Can you work these out from the model? Positions are in its coordinate system, mm. Face numbers are marked on the shaded views. A direction names the side the tool comes from. Give positions to 0.01 mm unless a question says otherwise; leave off trailing zeros. Order: outer loops, then holes, each group sorted by start corner. A loop starts at its lowest first (then second) coordinate and runs counter-clockwise, first axis right, second up.
Item 1: I want a section at B-B, the plane x = 0. Write out the boundary of the cut face in (y, z), then the cut area to 3 significant figures.
Item 2: Which directions (+Z, -Z, +X, -X, +Y, -Y) give clear straight access to the entire face, cutting with the end or side of a thin tool? Please do the marked faces 1, 2, 3 and 4.
Item 3: I'm going to push flat-ended pins straight in: pin 1 Ø1 at (x, y) = (1, 77.5) entering from -Z; pin 2 Ø4.5 at (x, y) = (0, 47) entering from -Z; pin 3 Ø3 at (x, z) = (1, -37.5) entering from +Y; pin 4 Ø3 at (x, y) = (-0.5, 33) entering from +Z. Where does each tip first touch, or does it pass through?
Item 4: I want a section at A-A, the plane y = 65.5. Write out the boundary of the cut face in (x, z).
Item 5: If I drill on line 1 along Z through (x, y) = (3.75, 36); line 2 along Y through (x, z) = (0, 30.9); line 3 along Y through (x, z) = (-2, -23.5), over which ranges is the centre line in solid material (lowest first)?
Item 6: I want a section at D-D, the plane z = 11. Write out the boundary of the cut face in (x, y), then the cut area to 3 significant figures.
Item 7: I want a section at C-C, the plane y = 47. Write out the boundary of the cut face in (x, z).
Item 8: If we mould it in two halves opening along Z, with no side actions, what happens to the marked faces 5, 6 and 7? For each: +Z half, -Z half, draft (parallel to the pull), parting line (faces both ways), or undercut.
```python
from build123d import *

# Parameters (mm, degrees)
BOSS_EXTRUDE1_DEPTH      = 5
BOSS_EXTRUDE1_DEPTH_BACK = 5
SKETCH2_R                = 2.5
CUT_EXTRUDE1_DEPTH       = 124.328828747


with BuildPart() as part:
    # Sketch1 → Boss-Extrude1 (new, two sides: drawn at the far end of the back side and taken through both)
    with BuildSketch(Plane(origin=(0, 0, 0), x_dir=(0, 0, -1), z_dir=(1, 0, 0)).offset(-BOSS_EXTRUDE1_DEPTH_BACK)):
        Polygon((-33, 3), (-33, 97), (33, 97), (33, 3), (43, 3), (43, 0), (33, 0), (28, 0), (28, 92), (-28, 92), (-28, 0), (-33, 0), (-43, 0), (-43, 3), align=None)
    extrude(amount=BOSS_EXTRUDE1_DEPTH + BOSS_EXTRUDE1_DEPTH_BACK)

    # Sketch2 → Cut-Extrude1 (cut, through all)
    with BuildSketch(Plane.XY.offset(33)):
        with Locations((0, 47)):
            Circle(SKETCH2_R)
    extrude(amount=-CUT_EXTRUDE1_DEPTH, mode=Mode.SUBTRACT)


solid = part.part
```
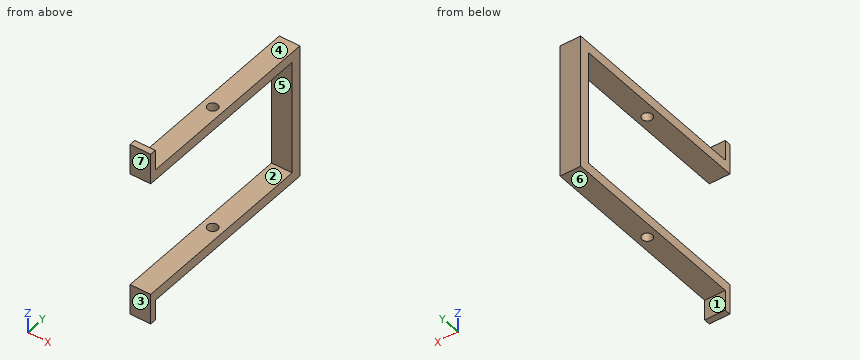
Results list:
1. outline: (0, -43) - (3, -43) - (3, -33) - (44.5, -33) - (44.5, -28) - (0, -28) - close; (0, 28) - (44.5, 28) - (44.5, 33) - (3, 33) - (3, 43) - (0, 43) - close; (49.5, -33) - (97, -33) - (97, 33) - (49.5, 33) - (49.5, 28) - (92, 28) - (92, -28) - (49.5, -28) - close
1. area: 1,260 mm2
2. face 1: -Z, +X, -X, +Y
2. face 2: +X, -X, -Y
2. face 3: +Z, -Z, +X, -X, -Y
2. face 4: +Z, +X, -X, +Y
3. pin 1: stops at z = -33
3. pin 2: passes through
3. pin 3: stops at y = 3
3. pin 4: stops at z = 33
4. outline: (-5, -33) - (5, -33) - (5, -28) - (-5, -28) - close; (-5, 28) - (5, 28) - (5, 33) - (-5, 33) - close
5. line 1: z = -33 to -28, 28 to 33
5. line 2: y = 0 to 44.5, 49.5 to 97
5. line 3: y = 92 to 97
6. outline: (-5, 92) - (5, 92) - (5, 97) - (-5, 97) - close
6. area: 50.0 mm2
7. outline: (-5, -33) - (-2.5, -33) - (-2.5, -28) - (-5, -28) - close; (-5, 28) - (-2.5, 28) - (-2.5, 33) - (-5, 33) - close; (2.5, -33) - (5, -33) - (5, -28) - (2.5, -28) - close; (2.5, 28) - (5, 28) - (5, 33) - (2.5, 33) - close
8. face 5: undercut
8. face 6: -Z half
8. face 7: draft
